```python
from build123d import *

# Parameters (mm, degrees)
BOSS_EXTRUDE1_DEPTH = 33
BOSS_EXTRUDE2_START = 32
BOSS_EXTRUDE2_DEPTH = 1
BOSS_EXTRUDE3_START = 33
SKETCH1_7_R         = 12
BOSS_EXTRUDE3_DEPTH = 1
CHAMFER1_SIZE       = 1
BOSS_EXTRUDE4_DEPTH = 10
BOSS_EXTRUDE5_START = 29
SKETCH1_9_W         = 2
SKETCH1_9_H         = 2
BOSS_EXTRUDE5_DEPTH = 4
BOSS_EXTRUDE6_START = 28
BOSS_EXTRUDE6_DEPTH = 5


with BuildPart() as part:
    # Sketch1 → Boss-Extrude1 (new body)
    with BuildSketch(Plane(origin=(0, 0, 0), x_dir=(1, 0, 0), z_dir=(0, 1, 0))):
        with BuildLine():
            ThreePointArc((7.383924434, -9.459263182), (8.859947089, -8.093289663), (10.087120501, -6.5))
            Line((10.087120501, -6.5), (9.182183836, -6.5))
            ThreePointArc((9.182183836, -6.5), (0, -11.25), (-9.182183836, -6.5))
            ThreePointArc((-9.182183836, -6.5), (-11.25, 0), (-9.182183836, 6.5))
            ThreePointArc((-9.182183836, 6.5), (0, 11.25), (9.182183836, 6.5))
            Line((9.182183836, 6.5), (10.087120501, 6.5))
            ThreePointArc((10.087120501, 6.5), (7.6512779, 9.244346732), (4.5, 11.124297731))
            ThreePointArc((4.5, 11.124297731), (0, 12), (-4.5, 11.124297731))
            ThreePointArc((-4.5, 11.124297731), (-10.392304845, 6), (-11.883924434, -1.665034548))
            ThreePointArc((-11.883924434, -1.665034548), (-10.392304845, -6), (-7.383924434, -9.459263182))
            ThreePointArc((-7.383924434, -9.459263182), (0, -12), (7.383924434, -9.459263182))
        make_face()
    extrude(amount=BOSS_EXTRUDE1_DEPTH)



with BuildPart() as body_2:
    # Sketch1<6> → Boss-Extrude2 (new body)
    with BuildSketch(Plane(origin=(0, 0, 0), x_dir=(1, 0, 0), z_dir=(0, 1, 0)).offset(BOSS_EXTRUDE2_START)):
        with BuildLine():
            ThreePointArc((10.087120501, -6.5), (11.248374399, -4.180200161), (11.883924434, -1.665034548))
            ThreePointArc((11.883924434, -1.665034548), (11.970945936, -0.834537834), (12, 0))
            ThreePointArc((12, 0), (11.511851415, 3.387813011), (10.087120501, 6.5))
            Line((10.087120501, 6.5), (9.182183836, 6.5))
            ThreePointArc((9.182183836, 6.5), (10.72058926, 3.410493501), (11.25, 0))
            ThreePointArc((11.25, 0), (10.72058926, -3.410493501), (9.182183836, -6.5))
            Line((9.182183836, -6.5), (10.087120501, -6.5))
        make_face()
    extrude(amount=BOSS_EXTRUDE2_DEPTH)


with BuildPart() as part_1:
    add(part.part)

    add(body_2.part)  # Boss-Extrude3 merges body 2
    # Sketch1<7> → Boss-Extrude3 (add)
    with BuildSketch(Plane(origin=(0, 0, 0), x_dir=(1, 0, 0), z_dir=(0, 1, 0)).offset(BOSS_EXTRUDE3_START)):
        with Locations(Location((0, 0, 0), (0, 0, 32.797168296))):
            Circle(SKETCH1_7_R)
    extrude(amount=BOSS_EXTRUDE3_DEPTH)

    # Chamfer1
    chamfer1_edges = [part_1.edges().sort_by_distance(p)[0] for p in [
        (-10.087120501, 34, 6.5),
    ]]
    chamfer(chamfer1_edges, length=CHAMFER1_SIZE - 0.0001)  # a hair under: the kernel refuses the full size

    # Sketch1<8> → Boss-Extrude4 (add)
    with BuildSketch(Plane(origin=(0, 0, 0), x_dir=(1, 0, 0), z_dir=(0, 1, 0))):
        with BuildLine():
            ThreePointArc((10.087120501, -6.5), (11.248374399, -4.180200161), (11.883924434, -1.665034548))
            ThreePointArc((11.883924434, -1.665034548), (11.970945936, -0.834537834), (12, 0))
            ThreePointArc((12, 0), (11.511851415, 3.387813011), (10.087120501, 6.5))
            Line((10.087120501, 6.5), (9.182183836, 6.5))
            ThreePointArc((9.182183836, 6.5), (10.72058926, 3.410493501), (11.25, 0))
            ThreePointArc((11.25, 0), (10.72058926, -3.410493501), (9.182183836, -6.5))
            Line((9.182183836, -6.5), (10.087120501, -6.5))
        make_face()
        with BuildLine():
            ThreePointArc((7.383924434, -9.459263182), (8.859947089, -8.093289663), (10.087120501, -6.5))
            Line((10.087120501, -6.5), (9.182183836, -6.5))
            ThreePointArc((9.182183836, -6.5), (0, -11.25), (-9.182183836, -6.5))
            ThreePointArc((-9.182183836, -6.5), (-11.25, 0), (-9.182183836, 6.5))
            ThreePointArc((-9.182183836, 6.5), (0, 11.25), (9.182183836, 6.5))
            Line((9.182183836, 6.5), (10.087120501, 6.5))
            ThreePointArc((10.087120501, 6.5), (7.6512779, 9.244346732), (4.5, 11.124297731))
            ThreePointArc((4.5, 11.124297731), (0, 12), (-4.5, 11.124297731))
            ThreePointArc((-4.5, 11.124297731), (-10.392304845, 6), (-11.883924434, -1.665034548))
            ThreePointArc((-11.883924434, -1.665034548), (-10.392304845, -6), (-7.383924434, -9.459263182))
            ThreePointArc((-7.383924434, -9.459263182), (0, -12), (7.383924434, -9.459263182))
        make_face()
    extrude(amount=BOSS_EXTRUDE4_DEPTH)

    # Sketch1<9> → Boss-Extrude5 (add)
    with BuildSketch(Plane(origin=(0, 0, 0), x_dir=(1, 0, 0), z_dir=(0, 1, 0)).offset(BOSS_EXTRUDE5_START)):
        with Locations((-5.154076544, -5.5)):
            Rectangle(SKETCH1_9_W, SKETCH1_9_H)
        with Locations((6.003328083, -5.5)):
            Rectangle(SKETCH1_9_W, SKETCH1_9_H)
        with Locations((6.003328083, 5.5)):
            Rectangle(SKETCH1_9_W, SKETCH1_9_H)
        with Locations((-5.154076544, 5.5)):
            Rectangle(SKETCH1_9_W, SKETCH1_9_H)
    extrude(amount=BOSS_EXTRUDE5_DEPTH)

    # Sketch1<11> → Boss-Extrude6 (add)
    with BuildSketch(Plane(origin=(0, 0, 0), x_dir=(1, 0, 0), z_dir=(0, 1, 0)).offset(BOSS_EXTRUDE6_START)):
        with BuildLine():
            ThreePointArc((-9.182183836, -6.5), (0, -11.25), (9.182183836, -6.5))
            Line((9.182183836, -6.5), (7.003328083, -6.5))
            Line((7.003328083, -6.5), (5.003328083, -6.5))
            Line((5.003328083, -6.5), (0, -6.5))
            Line((0, -6.5), (-4.154076544, -6.5))
            Line((-4.154076544, -6.5), (-6.154076544, -6.5))
            Line((-6.154076544, -6.5), (-9.182183836, -6.5))
        make_face()
        with BuildLine():
            Line((7.003328083, 6.5), (9.182183836, 6.5))
            ThreePointArc((9.182183836, 6.5), (0, 11.25), (-9.182183836, 6.5))
            Line((-9.182183836, 6.5), (-6.154076544, 6.5))
            Line((-6.154076544, 6.5), (-4.154076544, 6.5))
            Line((-4.154076544, 6.5), (0, 6.5))
            Line((0, 6.5), (5.003328083, 6.5))
            Line((5.003328083, 6.5), (7.003328083, 6.5))
        make_face()
    extrude(amount=BOSS_EXTRUDE6_DEPTH)


solid = part_1.part
```
For this review, take the finished solid that the model builds, in its own axes (mm). A direction names the side the tool comes from. Round coordinates to 2 decimals unless told otherwise and drop trailing zeros. Write each loop counter-clockwise with the first axis right and the second up, starting at its lowest first coordinate (ties: lowest second). Pieces come first, ordered by that corner, then holes. Notation, with made-up numbers: M 17,-29.75 L 73,-29.75 A19 ccw 73,-9.75 Z; hole C 81.5,48.5 d11. An arc over 180 degrees is marked long. One line per item, written item: value. Start each with the question number.
(1) The part is to be moulded in two halves that separate along Y. For faces 1 (the flat face through (-11, 0, 3)), 2 (the flat face through (1.9, 28.3, 6.5)), 3 (the flat face through (0, 34, 0)), 4 (the flat face through (-5, 31, 4.5)), say which applies: released by +Y, released by -Y, zero draft, split by the parting line, or undercut.
(2) Insertion check: pin 1 (1.6 mm diameter, centred on x = 6.5, z = 5.5, fed in from -Y); pin 2 (10 mm diameter, centred on x = 8, y = 4, fed in from +Z); pin 3 (2 mm diameter, centred on x = -5, y = 31.5, fed in from -Z). Each pin has a flat end and moves straight along its axis. Give the tip position at first contact, or say it passes through.
(3) We need section C-C (y = 27.5). Give the boundary of the cut face in (x, z).
(4) Machinability: for faces 5 (the flat face through (11.42, 32, -0.03)), 6 (the flat face through (-6.154, 31, 6)), 7 (the flat face through (6, 29, 5)), 8 (the flat face through (2, 29, -6.5)), which of the approach directions +Z, -Z, +X, -X, +Y, -Y give a long, thin tool a straight path to every point of the face, cutting with its end or side? Answer none if there is none.
(5) Wall thickness on line 1 (Z direction, x = 0.25, y = 19); line 2 (Y direction, x = -6, z = -0.5); line 3 (Z direction, x = 4.5, y = 15.5): over which ranges is each line inside the solid? List them lowest first.
(6) We need section A-A (y = 7). Give the boundary of the cut face in (x, z).
(7) We need section B-B (x = 0). Give the boundary of the cut face in (y, z), and give its area (3 significant figures).
Result:
1. face 1: released by -Y
1. face 2: undercut
1. face 3: released by +Y
1. face 4: zero draft
2. pin 1: y = 29
2. pin 2: z = 11.62
2. pin 3: z = -11.31
3. outline: M 9.18,-6.5 A11.25 cw long 9.18,6.5 L 10.09,6.5 A12 ccw long 10.09,-6.5 Z
4. face 5: +X
4. face 6: -Y
4. face 7: +X, -Y
4. face 8: none
5. line 1: -12 to -11.25, 11.25 to 12
5. line 2: 33 to 34
5. line 3: -11.12 to -10.31, 10.31 to 11.12
6. outline: C 0,0 d24; hole C 0,0 d22.5
7. outline: M 0,-12 L 33,-12 L 34,-11 L 34,11 L 33,12 L 0,12 L 0,11.25 L 28,11.25 L 28,6.5 L 33,6.5 L 33,-6.5 L 28,-6.5 L 28,-11.25 L 0,-11.25 Z
7. area: 120 mm²
